from build123d import *

# Parameters (mm, degrees)
F2_W            = 11.5754483268
F2_H            = 76.3443418741
F3_REACH        = 137.2178993172
F3_COPIES_COUNT = 8
F5_W            = 11.5754483268
F5_H            = 76.3443418741
F6_REACH        = 212.2178993172
F6_COPIES_COUNT = 10


# Not quite as in the source:
# - a pattern or mirror of a feature is missing from the dataset's text; its kind, count and spacing are read off the source's solid


with BuildPart() as f1:
    # F0 (on Front) → F1 (revolve)
    with BuildSketch(Plane.XZ):
        with BuildLine():
            Line((0, 5), (0, 0))
            Line((0, 0), (60, 0))
            Line((60, 0), (60, 96))
            Line((60, 96), (55, 96))
            Line((55, 96), (55, 5))
            Line((55, 5), (50, 5))
            Line((50, 5), (50, 96))
            Line((50, 96), (45, 96))
            Line((45, 96), (45, 10))
            ThreePointArc((45, 10), (43.5355339059, 6.4644660941), (40, 5))
            Line((40, 5), (0, 5))
        make_face()
    revolve(axis=Axis((0, 0, 2.5), (0, 0, 1)))

    f3_end = f1.faces().sort_by_distance((-50, 0, 50.5))[0]
    # F2 (on Front) → F3 (cut, up to a face of the model that its end follows)
    with BuildSketch(Plane.XZ):
        with Locations((0, 48)):
            Rectangle(F2_W, F2_H)
    f3_long = extrude(amount=F3_REACH, mode=Mode.PRIVATE)
    f3 = split(f3_long, bisect_by=f3_end, keep=Keep.BOTTOM, mode=Mode.PRIVATE)
    add(f3, mode=Mode.SUBTRACT)

    # F3_copies: F3 ×8 about axis
    f3_copies_axis = Axis((0, 0, 0), (0, 0, 1))
    for i in range(1, F3_COPIES_COUNT):
        add(f3.rotate(f3_copies_axis, i * 360 / F3_COPIES_COUNT), mode=Mode.SUBTRACT)

    f6_end = f1.faces().sort_by_distance((-55, 0, 50.5))[0]
    # F5 (on offset) → F6 (cut, up to a face of the model that its end follows)
    with BuildSketch(Plane.XZ.offset(75)):
        with Locations((0, 48)):
            Rectangle(F5_W, F5_H)
    f6_long = extrude(amount=-F6_REACH, mode=Mode.PRIVATE)
    f6 = split(f6_long, bisect_by=f6_end, keep=Keep.ALL, mode=Mode.PRIVATE).solids().sort_by_distance((0, -75, 48))[0]
    add(f6, mode=Mode.SUBTRACT)

    # F6_copies: F6 ×10 about axis
    f6_copies_axis = Axis((0, 0, 0), (0, 0, 1))
    for i in range(1, F6_COPIES_COUNT):
        add(f6.rotate(f6_copies_axis, i * 360 / F6_COPIES_COUNT), mode=Mode.SUBTRACT)


solid = f1.part
Read the model definition and answer for the solid it produces. Units are mm, in the model's axes. A direction names the side the tool comes from. Round coordinates to 2 decimals unless told otherwise and drop trailing zeros. Loops run counter-clockwise (first coordinate to the right, second up) from the corner with the lowest first, then second, coordinate; pieces in that order, holes last.
Q1. Section B-B on y = 0 is taken. Write down the section's boundary in (x, z).
Q2. Determine the mould class of faces 1 (the face through (1, 1, 0)), 2 (the face through (52.652, 23.193, 47.466)), 3 (the face through (-5.788, -47, 47)) for opening direction X: released by +X, released by -X, zero draft, split by the parting line, or undercut.
Q3. Which of the six approach directions +Z, -Z, +X, -X, +Y, -Y give full straight-line access (tool end or side, diameter ignored) to faces 4 (the face through (46.187, -19.15, 51.137)), 5 (the face through (0, -47, 9.828)), 6 (the face through (38.33, -42.91, 47.47)), 7 (the face through (-47, 0, 86.172))?
Q4. Section A-A on x = 0 is taken. Give the number of separate pieces and of enclosed holes in the cut face, and give its area (3 significant figures).
Q5. Consider probe 1 along X at (y, z) = (-6, 74); probe 2 along X at (y, z) = (30, 76.5); probe 3 along Y at (x, z) = (8, 28.5). Determine where each line is inside the solid, lowest interval first.
Q6. Each of these flat-tipped pins is pushed along its axis until it touches: pin 1 (2.5 mm diameter, centred on x = 46.5, z = 58, fed in from -Y); pin 2 (1 mm diameter, centred on y = -7.5, z = 48.5, fed in from -X); pin 3 (1 mm diameter, centred on y = -4, z = 71.5, fed in from +X). Where does it stop, or does it pass through?
Output:
1. outline: (-60, 0) - (60, 0) - (60, 96) - (55, 96) - (55, 5) - (50, 5) - (50, 9.83) - (45, 9.83) arc R5 cw to (40, 5) - (-40, 5) arc R5 cw to (-45, 9.83) - (-50, 9.83) - (-50, 5) - (-55, 5) - (-55, 96) - (-60, 96) - close; (-50, 86.17) - (-45, 86.17) - (-45, 96) - (-50, 96) - close; (45, 86.17) - (50, 86.17) - (50, 96) - (45, 96) - close
2. face 1: zero draft
2. face 2: released by +X
2. face 3: undercut
3. face 4: +Z
3. face 5: +Y, -Y
3. face 6: -Y
3. face 7: none
4. separate pieces: 5
4. enclosed holes: 0
4. area: 904 mm2
5. probe 1: x = -59.7 to -54.67, -49.64 to -44.6, 44.6 to 49.64, 54.67 to 59.7
5. probe 2: x = -51.96 to -46.1, -40 to -38.19, 38.19 to 40, 46.1 to 51.96
5. probe 3: y = -59.46 to -54.42, -49.36 to -44.28, 44.28 to 49.36, 54.42 to 59.46
6. pin 1: stops at y = -39.4
6. pin 2: stops at x = -59.59
6. pin 3: stops at x = 59.9
